Geometry check sheet. Reference: drawing and pictorial views, mm from the part's lowest x, y, z. A direction names the side the tool comes from. Coordinates: 2 decimals unless noted, no trailing zeros. Loops run counter-clockwise (first coordinate to the right, second up) from the corner with the lowest first, then second, coordinate; pieces in that order, holes last. Notation, with made-up numbers: (-23, 52.5) -> (-9, 52.5) arc R23 ccw to (-9, 62.5) -> close; hole circle Ø7 at (85.25, 52). An arc over 180 degrees is marked (long way). Answer as a JSON object with one key per item and string values.
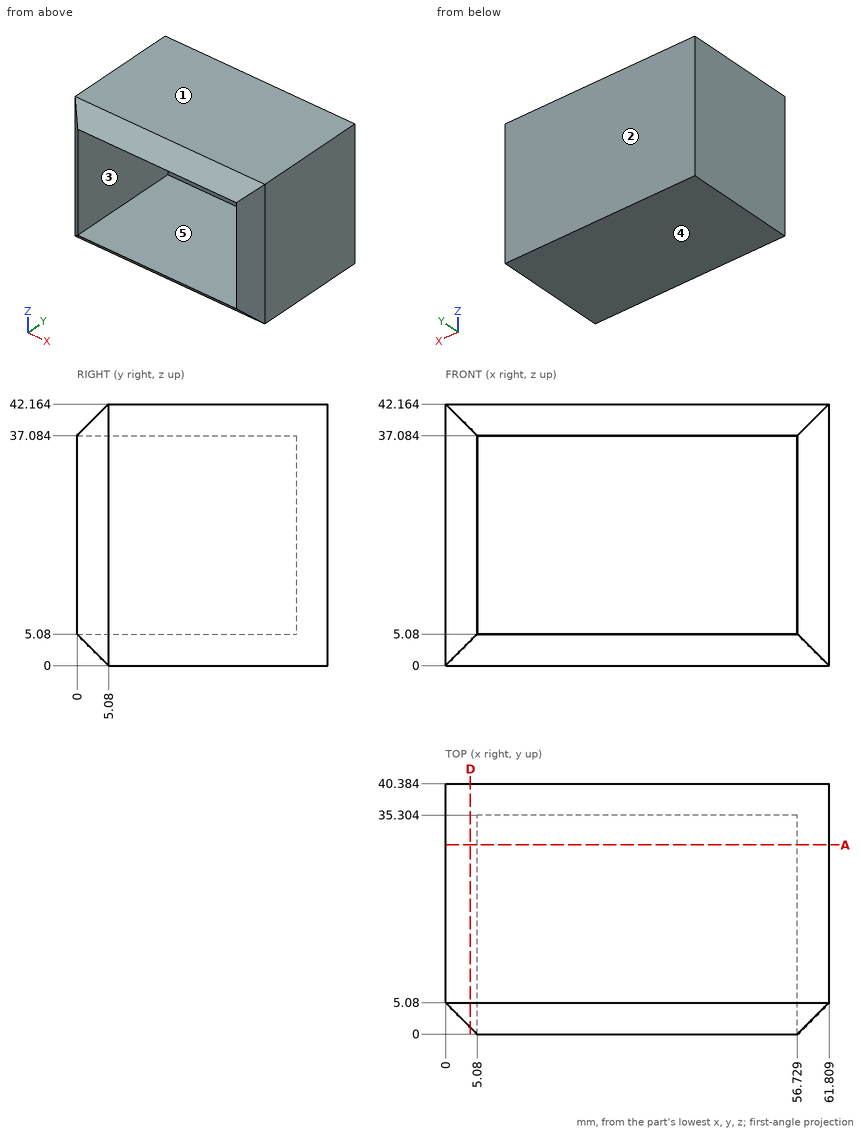
1. Mould release check, pull along Z, two halves, no side actions. Record for the marked faces 1, 2 and 3: released by +Z, released by -Z, zero draft, split by the parting line, or undercut.
Evaluation:
{"face 1": "released by +Z", "face 2": "zero draft", "face 3": "undercut"}
2. Depth check by flat-ended pin: P1, Ø3, axis at x = 31.5, z = 12.5, coming from the -Y side; P2, Ø6, axis at x = 13, z = 36.5, coming from the -Y side. Enter the tip coordinate at first touch or a pass-through.
Evaluation:
{"P1": "stops at y = 35.3", "P2": "stops at y = 0"}
3. Section check A-A, the plane y = 30.5. Record the boundary of the cut face in (x, z), then the cut area to 3 significant figures.
Evaluation:
{"outline": "(0, 0) -> (61.81, 0) -> (61.81, 42.16) -> (0, 42.16) -> close; hole (5.08, 5.08) -> (56.73, 5.08) -> (56.73, 37.08) -> (5.08, 37.08) -> close", "area": "953 mm^2"}
4. Thickness scan on probe 1 along X at (y, z) = (11, 28.5); probe 2 along Z at (x, y) = (34, 29); probe 3 along Y at (x, z) = (23, 13.5). Record the ranges inside material, lowest first. Write a range as from..to.
Evaluation:
{"probe 1": "x = 0..5.08, 56.73..61.81", "probe 2": "z = 0..5.08, 37.08..42.16", "probe 3": "y = 35.3..40.38"}
5. Section check D-D, the plane x = 4. Record the boundary of the cut face in (y, z).
Evaluation:
{"outline": "(1.08, 4) -> (5.08, 0) -> (40.38, 0) -> (40.38, 42.16) -> (5.08, 42.16) -> (1.08, 38.16) -> close"}
6. Tool access check on the marked faces 4 and 5. Record the directions out of +Z, -Z, +X, -X, +Y, -Y that give a thin tool (end or side, any length) a straight path to the whole face; none if there is none.
Evaluation:
{"face 4": "-Z, +X, -X, +Y, -Y", "face 5": "-Y"}
